For this review, take the finished solid that the model builds, in its own axes (mm). Give positions to 0.01 mm unless a question says otherwise; leave off trailing zeros. Order: outer loops, then holes, each group sorted by start corner. A loop starts at its lowest first (then second) coordinate and runs counter-clockwise, first axis right, second up. Notation, with made-up numbers: (39, 75) -> (56, 75) arc R24 ccw to (56, 91) -> close; hole circle Ø4 at (41.25, 53). An arc over 180 degrees is marked (long way). Return JSON: item names as keys, results as strings. Group by question number.
1) Add section A-A (x = -6). Give the boundary of the cut face in (y, z), then the cut area to 3 significant figures.
2) Add section C-C (z = 0.65). State how many separate pieces and enclosed holes the cut face has, then the cut area to 3 significant figures.
3) Add section B-B (y = -46). Give the boundary of the cut face in (x, z), then the cut area to 3 significant figures.
4) To check wall thickness, follow line 1 along X through (y, z) = (140, 1.2); line 2 along Y through (x, z) = (-150, 2.4); line 3 along X through (y, z) = (-1.5, 0.95). State the ranges of each line that lie inside material, in increasing order.
from build123d import *

# Parameters (mm, degrees)
SKETCH_W        = 400
SKETCH_H        = 380
PAD_DEPTH       = 3
SKETCH001_R     = 2
POCKET_DEPTH    = 3.001
POCKET001_DEPTH = 3.001
SKETCH003_R     = 3
SKETCH003_R_2   = 5.5
POCKET002_DEPTH = 3.001
FILLET_R        = 30.16
SKETCH004_W     = 44
SKETCH004_H     = 44
POCKET003_DEPTH = 3.001
FILLET001_R     = 3


with BuildPart() as part:
    # Sketch → Pad (new body)
    with BuildSketch(Plane.XY):
        Rectangle(SKETCH_W, SKETCH_H)
    extrude(amount=PAD_DEPTH)

    # Sketch001 (on Face6 of Pad) → Pocket (cut, through all)
    with BuildSketch(Plane.XY.offset(3)):
        with Locations((-150, 175)):
            Circle(SKETCH001_R)
        with Locations((-185, 140)):
            Circle(SKETCH001_R)
        with Locations((-185, -140)):
            Circle(SKETCH001_R)
        with Locations((-150, -175)):
            Circle(SKETCH001_R)
        with Locations((150, -175)):
            Circle(SKETCH001_R)
        with Locations((185, -140)):
            Circle(SKETCH001_R)
        with Locations((185, 140)):
            Circle(SKETCH001_R)
        with Locations((150, 175)):
            Circle(SKETCH001_R)
    extrude(amount=-POCKET_DEPTH, mode=Mode.SUBTRACT)

    # Sketch002 (on Face5 of Pocket) → Pocket001 (cut, through all)
    with BuildSketch(Plane.XY.offset(3)):
        with BuildLine():
            Line((-150, 150), (150, 150))
            ThreePointArc((160, 140), (157.071068, 147.071068), (150, 150))
            Line((160, 140), (160, -140))
            ThreePointArc((150, -150), (157.071068, -147.071068), (160, -140))
            Line((150, -150), (-150, -150))
            ThreePointArc((-160, -140), (-157.071068, -147.071068), (-150, -150))
            Line((-160, -140), (-160, 140))
            ThreePointArc((-150, 150), (-157.071068, 147.071068), (-160, 140))
        make_face()
    extrude(amount=-POCKET001_DEPTH, mode=Mode.SUBTRACT)

    # Sketch003 (on Face5 of Pocket001) → Pocket002 (cut, through all)
    with BuildSketch(Plane.XY.offset(3)):
        with Locations((-135.5, 157.5)):
            Circle(SKETCH003_R)
        with Locations((-110.5, 160)):
            Circle(SKETCH003_R_2)
    extrude(amount=-POCKET002_DEPTH, mode=Mode.SUBTRACT)

    # Fillet
    fillet_edges = [part.edges().sort_by_distance(p)[0] for p in [
        (-200, -190, 1.5),
        (-200, 190, 1.5),
        (200, 190, 1.5),
        (200, -190, 1.5),
    ]]
    fillet(fillet_edges, radius=FILLET_R)

    # Sketch004 (on Face5 of Fillet) → Pocket003 (cut, through all)
    with BuildSketch(Plane.XY.offset(3)):
        with Locations((0, 143)):
            Rectangle(SKETCH004_W, SKETCH004_H)
    extrude(amount=-POCKET003_DEPTH, mode=Mode.SUBTRACT)

    # Fillet001
    fillet001_edges = [part.edges().sort_by_distance(p)[0] for p in [
        (-22, 165, 1.5),
        (22, 165, 1.5),
    ]]
    fillet(fillet001_edges, radius=FILLET001_R)


solid = part.part
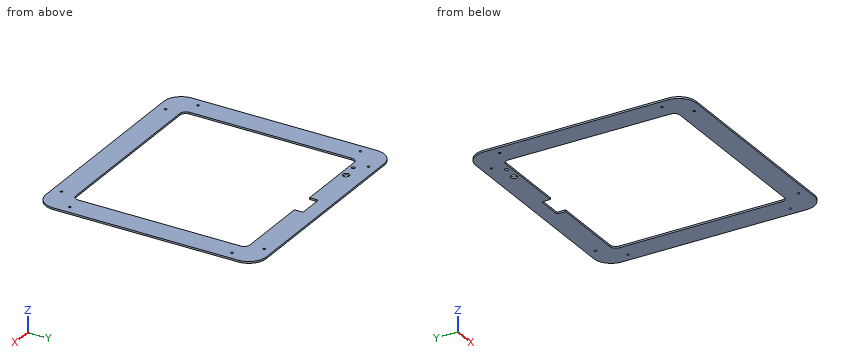
Evaluation:
{
 "1": {"outline": "(-190, 0) -> (-150, 0) -> (-150, 3) -> (-190, 3) -> close; (165, 0) -> (190, 0) -> (190, 3) -> (165, 3) -> close", "area": "195 mm^2"},
 "2": {"separate pieces": "1", "enclosed holes": "11", "area": "54,400 mm^2"},
 "3": {"outline": "(-200, 0) -> (-160, 0) -> (-160, 3) -> (-200, 3) -> close; (160, 0) -> (200, 0) -> (200, 3) -> (160, 3) -> close", "area": "240 mm^2"},
 "4": {"line 1": "-200 to -187, -183 to -160, 160 to 183, 187 to 200", "line 2": "-190 to -177, -173 to -150, 150 to 173, 177 to 190", "line 3": "-200 to -160, 160 to 200"}
}
